Autodesk Inventor part; units mm, degrees
ref_plane "YZ Plane" through (0, 0, 0) normal (1, 0, 0) x (0, 1, 0)
ref_plane "XZ Plane" through (0, 0, 0) normal (0, 1, 0) x (-1, 0, 0)
ref_plane "XY Plane" through (0, 0, 0) normal (0, 0, 1) x (1, 0, 0)
sketch "Sketch1" plane through (0, 0, 0) normal (0, 0, 1) x (1, 0, 0)
  line L0 (0, 0) -> (-65.1047, 320)
  line L1 (-65.1047, 320) -> (375, 320)
  line L2 (375, 320) -> (375, 0)
  line L3 (375, 0) -> (0, 0)
  dimension "d0" = 320
  dimension "d1" = 78.5
  dimension "d2" = 375
extrude "Extrusion1" add sketch "Sketch1" along normal blind 5
sketch "Sketch2" plane through (0, 0, 5) normal (0, 0, 1) x (1, 0, 0)
  line L0 (0, 0) -> (375, 0)
  point P0 (190, 290)
  point P1 (190, 270)
  point P2 (95, 165)
  point P3 (95, 145)
  point P4 (285, 165)
  point P5 (285, 145)
  point P6 (30, 50)
  point P7 (30, 30)
  point P8 (160, 50)
  point P9 (160, 30)
  point P10 (220, 50)
  point P11 (220, 30)
  point P12 (350, 50)
  point P13 (350, 30)
  point P14 (190, 315)
  point P15 (30, 5)
  point P16 (160, 5)
  point P17 (220, 5)
  point P18 (350, 5)
  dimension "d5" = 20
  dimension "d6" = 20
  dimension "d7" = 20
  dimension "d15" = 25
  dimension "d16" = 105
  dimension "d17" = 95
  dimension "d19" = 25
  dimension "d20" = 5
  dimension "d21" = 30
  dimension "d29" = 60
  dimension "d30" = 130
  dimension "d31" = 130
  dimension "d32" = 65
  dimension "d33" = 65
  dimension "d35" = 190
  dimension "d36" = 95
hole "Hole1" at (190, 290, 5) at (190, 270, 5) at (95, 165, 5) at (95, 145, 5) at (285, 165, 5) at (285, 145, 5) at (30, 50, 5) at (30, 30, 5) at (160, 50, 5) at (160, 30, 5) at (220, 50, 5) at (220, 30, 5) at (350, 50, 5) at (350, 30, 5) at (190, 315, 5) at (30, 5, 5) at (160, 5, 5) at (220, 5, 5) at (350, 5, 5) direction (0, 0, -1) diameter 4.5 end through all
sketch "Sketch3" plane through (0, 0, 5) normal (0, 0, 1) x (1, 0, 0)
  circle A0 centre (220, 5) radius 2.25
  circle A1 centre (30, 5) radius 2.25
  circle A2 centre (220, 30) radius 2.25
  circle A3 centre (160, 30) radius 2.25
  circle A4 centre (30, 30) radius 2.25
  circle A5 centre (285, 145) radius 2.25
  circle A6 centre (95, 145) radius 2.25
  circle A7 centre (190, 270) radius 2.25
  circle A8 centre (190, 290) radius 2.25
  circle A9 centre (95, 165) radius 2.25
  circle A10 centre (285, 165) radius 2.25
  circle A11 centre (30, 50) radius 2.25
  circle A12 centre (160, 50) radius 2.25
  circle A13 centre (220, 50) radius 2.25
  circle A14 centre (160, 5) radius 2.25
  line L0 (-65.1047, 320) -> (0, 0)
  line L1 (0, 0) -> (375, 0)
  line L2 (375, 0) -> (375, 320)
  line L3 (375, 320) -> (-65.1047, 320)
  point P0 (190, 210)
  point P1 (95, 85)
  point P2 (285, 85)
  dimension "d37" = 60
  dimension "d38" = 60
hole "Hole2" at (190, 210, 5) at (95, 85, 5) at (285, 85, 5) direction (0, 0, -1) diameter 7 end through all
sketch "Sketch4" plane through (0, 0, 5) normal (0, 0, 1) x (1, 0, 0)
  circle A0 centre (95, 85) radius 3.5
  circle A1 centre (190, 210) radius 3.5
  circle A2 centre (285, 85) radius 3.5
  circle A3 centre (220, 5) radius 2.25
  circle A4 centre (30, 5) radius 2.25
  circle A5 centre (220, 30) radius 2.25
  circle A6 centre (160, 30) radius 2.25
  circle A7 centre (30, 30) radius 2.25
  circle A8 centre (285, 145) radius 2.25
  circle A9 centre (95, 145) radius 2.25
  circle A10 centre (190, 270) radius 2.25
  circle A11 centre (190, 290) radius 2.25
  circle A12 centre (95, 165) radius 2.25
  circle A13 centre (285, 165) radius 2.25
  circle A14 centre (30, 50) radius 2.25
  circle A15 centre (160, 50) radius 2.25
  circle A16 centre (220, 50) radius 2.25
  circle A17 centre (160, 5) radius 2.25
  line L0 (-65.1047, 320) -> (0, 0)
  line L1 (0, 0) -> (375, 0)
  line L2 (375, 0) -> (375, 320)
  line L3 (375, 320) -> (-65.1047, 320)
  point P0 (215, 185)
  point P1 (165, 185)
  point P2 (70, 60)
  point P3 (120, 60)
  point P4 (260, 60)
  point P5 (310, 60)
  dimension "d46" = 25
  dimension "d47" = 25
  dimension "d48" = 50
  dimension "d49" = 50
  dimension "d50" = 25
  dimension "d51" = 50
  dimension "d52" = 25
  dimension "d53" = 25
hole "Hole3" at (215, 185, 5) at (165, 185, 5) at (70, 60, 5) at (120, 60, 5) at (260, 60, 5) at (310, 60, 5) direction (0, 0, -1) diameter 3.4 end through all
chamfer "Chamfer1" distance 150 angle 45 1 edges at (375, 320, 2.5)
sketch "Sketch5" plane through (0, 0, 5) normal (0, 0, 1) x (1, 0, 0)
  line L0 (-65.1047, 320) -> (0, 0)
  line L1 (225, 320) -> (-65.1047, 320)
  line L2 (0, 0) -> (375, 0)
  point P0 (-35.0552, 235)
  point P1 (-5.15, 88.0113)
  dimension "d64" = 12.5
  dimension "d65" = 12.5
  dimension "d66" = 150
  dimension "d67" = 85
  dimension "d68" = 88.0113
hole "Hole4" at (-35.0552, 235, 5) at (-5.15, 88.0113, 5) direction (0, 0, -1) diameter 4.5 end through all
sketch "Sketch6" plane through (0, 0, 5) normal (0, 0, 1) x (1, 0, 0)
  circle A0 centre (-35.0552, 235) radius 2.25
  circle A1 centre (-5.15, 88.0113) radius 2.25
  line L0 (225, 320) -> (375, 170)
  line L1 (225, 320) -> (-65.1047, 320)
  line L2 (-65.1047, 320) -> (0, 0)
  line L3 (0, 0) -> (375, 0)
  line L4 (375, 0) -> (375, 170)
  circle A2 centre (260, 60) radius 1.7
  circle A3 centre (70, 60) radius 1.7
  circle A4 centre (215, 185) radius 1.7
  circle A5 centre (165, 185) radius 1.7
  circle A6 centre (120, 60) radius 1.7
  circle A7 centre (310, 60) radius 1.7
  circle A8 centre (95, 85) radius 3.5
  circle A9 centre (190, 210) radius 3.5
  circle A10 centre (285, 85) radius 3.5
  circle A11 centre (220, 5) radius 2.25
  circle A12 centre (30, 5) radius 2.25
  circle A13 centre (350, 30) radius 2.25
  circle A14 centre (220, 30) radius 2.25
  circle A15 centre (160, 30) radius 2.25
  circle A16 centre (30, 30) radius 2.25
  circle A17 centre (285, 145) radius 2.25
  circle A18 centre (95, 145) radius 2.25
  circle A19 centre (190, 270) radius 2.25
  circle A20 centre (190, 290) radius 2.25
  circle A21 centre (95, 165) radius 2.25
  circle A22 centre (285, 165) radius 2.25
  circle A23 centre (30, 50) radius 2.25
  circle A24 centre (160, 50) radius 2.25
  circle A25 centre (220, 50) radius 2.25
  circle A26 centre (350, 50) radius 2.25
  circle A27 centre (190, 315) radius 2.25
  circle A28 centre (160, 5) radius 2.25
  circle A29 centre (350, 5) radius 2.25
  point P0 (125.4041, 180)
  point P1 (145, 184)
  point P2 (235, 184)
  point P3 (254.5959, 180)
  dimension "d76" = 20
  dimension "d77" = 4
  dimension "d78" = 20
  dimension "d79" = 45
  dimension "d80" = 26
  dimension "d81" = 45
hole "Hole5" at (125.4041, 180, 5) at (145, 184, 5) at (235, 184, 5) at (254.5959, 180, 5) direction (0, 0, -1) diameter 3.4 end through all
properties part number "Top_Separator Backboard" material "PMMA Plastic"
Here's how the part is built. I have some questions about the finished solid (model axes, mm). Round coordinates to 2 decimals unless told otherwise and drop trailing zeros. Order: outer loops, then holes, each group sorted by start corner. A loop starts at its lowest first (then second) coordinate and runs counter-clockwise, first axis right, second up. Notation, with made-up numbers: (-30, 47.25) -> (5, 47.25) arc R12 cw to (5, 57.25) -> close; hole circle Ø9 at (22, -37). An arc over 180 degrees is marked (long way). Return JSON: item names as keys, results as strings.
Q1. I need wall thicknesses on line 1 along Y through (x, z) = (95, 2.9); line 2 along Y through (x, z) = (30, 1.25); line 3 along X through (y, z) = (60, 3.85). Which ranges of each line are inside material? Lowest first, please. Write a range as from..to.
Filled sheet:
{"line 1": "y = 0..81.5, 88.5..142.75, 147.25..162.75, 167.25..320", "line 2": "y = 0..2.75, 7.25..27.75, 32.25..47.75, 52.25..320", "line 3": "x = -12.21..68.3, 71.7..118.3, 121.7..258.3, 261.7..308.3, 311.7..375"}
Q2. If we section it at A-A on x = 322: List the corners of the cut face in (y, z) for me.
Filled sheet:
{"outline": "(0, 0) -> (223, 0) -> (223, 5) -> (0, 5) -> close"}
Q3. If we section it at C-C on y = 198: List the corners of the cut face in (x, z) for me, plus the area to 3 significant figures.
Filled sheet:
{"outline": "(-40.28, 0) -> (347, 0) -> (347, 5) -> (-40.28, 5) -> close", "area": "1,940 mm^2"}
Q4. For pin 1 Ø1.5 at (y, z) = (184, 2) entering from +X; pin 2 Ø2.5 at (x, y) = (30, 30) entering from -Z; pin 3 Ø2 at (x, z) = (282.5, 0.5) entering from +Y, each with a flat end and sliding along its axis, tell me the tip position at first contact or that it passes through.
Filled sheet:
{"pin 1": "stops at x = 361.75", "pin 2": "passes through", "pin 3": "stops at y = 263.5"}
Q5. If we section it at B-B on z = 1.7: Give the number of separate pieces and of enclosed holes in the cut face, plus the area to 3 significant figures.
Filled sheet:
{"separate pieces": "1", "enclosed holes": "34", "area": "119,000 mm^2"}
